Part model, mm, in its own coordinate system. A direction names the side the tool comes from. Coordinates: 2 decimals unless noted, no trailing zeros. Loops run counter-clockwise (first coordinate to the right, second up) from the corner with the lowest first, then second, coordinate; pieces in that order, holes last. Notation, with made-up numbers: (-16, 36.25) -> (30, 36.25) arc R34 cw to (30, 69.25) -> close; hole circle Ø10 at (-26.5, -7.75). An arc over 180 degrees is marked (long way). One line per question, with ' | ' between items. Start each with the question number.
1) Cut at D-D (y = 3.25). List the corners of the cut face in (x, z), plus the area to 3 significant figures.
2) Cut at A-A (z = 10). List the corners of the cut face in (x, y).
3) Drop flat-ended pins along their axis: pin 1 (2 mm diameter, centred on y = 6, z = 5, fed in from -X); pin 2 (3 mm diameter, centred on y = 10.5, z = 5.5, fed in from +X); pin 3 (7.5 mm diameter, centred on y = 10, z = 10, fed in from -X); pin 4 (3 mm diameter, centred on x = 15, z = 10, fed in from +Y). Give the stop position or say it passes through.
4) Cut at C-C (x = 15). List the corners of the cut face in (y, z).
5) 3-axis set-ups, long thin cutter, end or side, ignore diameter. For faces 1 (the face through (9.87, 6.25, 10.05)), 2 (the face through (0.57, 0.6, 3.8)), 3 (the face through (25, 3, 10)), 4 (the face through (0, 12.98, 0.38)), 5 (the face through (16, 7, 4)): which of +Z, -Z, +X, -X, +Y, -Y reach the whole face in a straight line?
6) Cut at B-B (y = 10). List the corners of the cut face in (x, z).
7) Probe L1, parallel to Z at x = 15, y = 1.5; L2, parallel to Y at x = 3.75, z = 10; L3, parallel to X at y = 3, z = 10. List the from-to ranges inside material, lowest first. Write a range as from..to.
8) Two-plate mould, pull along X, no slides. Class faces 6 (the face through (0.57, 0.185, 12.835)), 7 (the face through (12.907, 3.549, 9.047)), 8 (the face through (10, 6, 20)): released by +X, released by -X, zero draft, split by the parting line, or undercut.
from build123d import *

# Parameters (mm, degrees)
AUFSATZ_LINEAR_AUSTRAGEN1_DEPTH      = 20
AUFSATZ_LINEAR_AUSTRAGEN2_DEPTH      = 20
AUFSATZ_LINEAR_AUSTRAGEN3_DEPTH      = 25
SCHNITT_LINEAR_AUSTRAGEN1_DEPTH      = 20
SCHNITT_LINEAR_AUSTRAGEN1_DEPTH_BACK = 20
SKIZZE2_R                            = 2.3
SKIZZE3_R                            = 3.75
SCHNITT_LINEAR_AUSTRAGEN2_DEPTH      = 34.526109228
SKIZZE4_R                            = 2.3
SCHNITT_LINEAR_AUSTRAGEN3_DEPTH      = 20
FASE1_SIZE                           = 0.75
VERRUNDUNG1_R                        = 2
SKIZZE7_R                            = 4.15
SCHNITT_LINEAR_AUSTRAGEN4_DEPTH      = 20
SKIZZE8_R                            = 4.15
SCHNITT_LINEAR_AUSTRAGEN5_DEPTH      = 20
VERRUNDUNG2_R                        = 1


with BuildPart() as part:
    # Skizze1 → Aufsatz-Linear austragen1 (new body)
    with BuildSketch(Plane.XY):
        Polygon((0, 0), (0, 20), (7, 20), (7, 7), (25, 7), (25, 0), align=None)
    extrude(amount=AUFSATZ_LINEAR_AUSTRAGEN1_DEPTH)

    # Skizze5 → Aufsatz-Linear austragen2 (add)
    with BuildSketch(Plane(origin=(0, 0, 0), x_dir=(-1, 0, 0), z_dir=(0, 0, -1))):
        Polygon((0, 6.5), (0, 13.5), (0.75, 12.75), (0.75, 7.25), align=None)
    extrude(amount=-AUFSATZ_LINEAR_AUSTRAGEN2_DEPTH)

    # Skizze6 → Aufsatz-Linear austragen3 (add)
    with BuildSketch(Plane.ZY):
        Polygon((6.5, 0), (13.5, 0), (12.75, -0.75), (7.25, -0.75), align=None)
    extrude(amount=-AUFSATZ_LINEAR_AUSTRAGEN3_DEPTH)

    # Skizze2 → Schnitt-Linear austragen1 (cut, two sides: drawn at the far end of the back side and taken through both)
    with BuildSketch(Plane.ZY.offset(-SCHNITT_LINEAR_AUSTRAGEN1_DEPTH_BACK)):
        with Locations(Location((10, 10, 0), (0, 0, 270))):
            Circle(SKIZZE2_R)
    extrude(amount=SCHNITT_LINEAR_AUSTRAGEN1_DEPTH + SCHNITT_LINEAR_AUSTRAGEN1_DEPTH_BACK, mode=Mode.SUBTRACT)

    # Skizze3 → Schnitt-Linear austragen2 (cut, through all)
    with BuildSketch(Plane(origin=(7, 0, 0), x_dir=(0, 0, -1), z_dir=(1, 0, 0))):
        with Locations((-10, 10)):
            Circle(SKIZZE3_R)
    extrude(amount=SCHNITT_LINEAR_AUSTRAGEN2_DEPTH, mode=Mode.SUBTRACT)

    # Skizze4 → Schnitt-Linear austragen3 (cut)
    with BuildSketch(Plane(origin=(0, 7, 0), x_dir=(1, 0, 0), z_dir=(0, 1, 0))):
        with Locations(Location((15, -10, 0), (0, 0, 258.031254445))):
            Circle(SKIZZE4_R)
    extrude(amount=-SCHNITT_LINEAR_AUSTRAGEN3_DEPTH, mode=Mode.SUBTRACT)

    # Fase1
    fase1_edges = [part.edges().sort_by_distance(p)[0] for p in [
        (0, 20, 10),
        (7, 20, 10),
        (7, 7, 16.125),
        (25, 7, 16.125),
        (25, 0, 16.75),
        (16, 7, 20),
        (7, 13.5, 20),
        (0, 3.25, 0),
        (0, 3.25, 20),
        (3.5, 20, 20),
        (-0.375, 6.875, 20),
        (-0.375, 13.125, 20),
        (-0.75, 10, 20),
        (-0.375, 6.875, 0),
        (-0.75, 10, 0),
        (-0.375, 13.125, 0),
        (0, 16.75, 20),
        (25, 0, 3.25),
        (25, -0.375, 13.125),
        (25, -0.75, 10),
        (25, -0.375, 6.875),
        (12.5, 0, 20),
        (7, 7, 3.875),
        (25, 7, 3.875),
        (25, 6.25, 10),
        (0, 16.75, 0),
        (3.5, 20, 0),
        (7, 13.5, 0),
        (16, 7, 0),
        (25, 3.5, 0),
        (12.5, 0, 0),
        (25, 3.5, 20),
    ]]
    chamfer(fase1_edges, length=FASE1_SIZE)

    # Verrundung1
    verrundung1_edges = [part.edges().sort_by_distance(p)[0] for p in [
        (0, 0, 3.625),
        (0, -0.375, 13.125),
        (0, -0.375, 6.875),
        (0, -0.75, 10),
        (0, 0, 16.375),
    ]]
    fillet(verrundung1_edges, radius=VERRUNDUNG1_R)

    # Skizze7 → Schnitt-Linear austragen4 (cut)
    with BuildSketch(Plane.ZY):
        with Locations((10, 10)):
            Circle(SKIZZE7_R)
    extrude(amount=SCHNITT_LINEAR_AUSTRAGEN4_DEPTH, mode=Mode.SUBTRACT)

    # Skizze8 → Schnitt-Linear austragen5 (cut)
    with BuildSketch(Plane.XZ):
        with Locations((15, 10)):
            Circle(SKIZZE8_R)
    extrude(amount=SCHNITT_LINEAR_AUSTRAGEN5_DEPTH, mode=Mode.SUBTRACT)

    # Verrundung2
    # the kernel refuses this fillet: 1 mm, written as the material it takes off along each edge
    with BuildSketch(Plane(origin=(15, -0.75, 10), x_dir=(-0.259943773458836, 0, -0.9656237541817109), z_dir=(0.9656237541817109, 0, -0.259943773458836))) as verrundung2_piece_1:
        with BuildLine():
            CenterArc((5.118245837, 1), VERRUNDUNG2_R, 194.477512186, 75.522487814)
            Line((4.15, 0.75), (4.130635083, 0.745))
            ThreePointArc((4.130635083, 0.745), (4.13, 0.375), (4.13, 0))
            Line((4.13, 0), (4.15, -0.02))
            Line((4.15, -0.02), (5.118245837, -0.02))
            Line((5.118245837, -0.02), (5.118245837, 0))
        make_face()
    revolve(axis=Axis((15, -0.75, 10), (0, 1, 0)), revolution_arc=149.866548224, mode=Mode.SUBTRACT)
    with BuildSketch(Plane(origin=(15, -0.75, 10), x_dir=(0.259943773458836, 0, -0.9656237541817109), z_dir=(-0.9656237541817109, 0, -0.259943773458836))) as verrundung2_piece_2:
        with BuildLine():
            CenterArc((5.118245837, -1), VERRUNDUNG2_R, 90, 75.522487814)
            Line((4.15, -0.75), (4.130635083, -0.745))
            ThreePointArc((4.130635083, -0.745), (4.13, -0.375), (4.13, 0))
            Line((4.13, 0), (4.15, 0.02))
            Line((4.15, 0.02), (5.118245837, 0.02))
            Line((5.118245837, 0.02), (5.118245837, 0))
        make_face()
    revolve(axis=Axis((15, -0.75, 10), (0, -1, 0)), revolution_arc=149.866548224, mode=Mode.SUBTRACT)
    with BuildSketch(Plane(origin=(-0.75, 10, 10), x_dir=(0, -0.9656237541817109, -0.2599437734588364), z_dir=(0, -0.2599437734588364, 0.9656237541817109))) as verrundung2_piece_3:
        with BuildLine():
            CenterArc((5.118245837, 1), VERRUNDUNG2_R, 194.477512186, 75.522487814)
            Line((4.15, 0.75), (4.130635083, 0.745))
            ThreePointArc((4.130635083, 0.745), (4.13, 0.375), (4.13, 0))
            Line((4.13, 0), (4.15, -0.02))
            Line((4.15, -0.02), (5.118245837, -0.02))
            Line((5.118245837, -0.02), (5.118245837, 0))
        make_face()
    revolve(axis=Axis((-0.75, 10, 10), (1, 0, 0)), revolution_arc=149.866548224, mode=Mode.SUBTRACT)
    with BuildSketch(Plane(origin=(-0.75, 10, 10), x_dir=(0, -0.9656237541817109, 0.2599437734588359), z_dir=(0, -0.2599437734588359, -0.9656237541817109))) as verrundung2_piece_4:
        with BuildLine():
            CenterArc((5.118245837, -1), VERRUNDUNG2_R, 90, 75.522487814)
            Line((4.15, -0.75), (4.130635083, -0.745))
            ThreePointArc((4.130635083, -0.745), (4.13, -0.375), (4.13, 0))
            Line((4.13, 0), (4.15, 0.02))
            Line((4.15, 0.02), (5.118245837, 0.02))
            Line((5.118245837, 0.02), (5.118245837, 0))
        make_face()
    revolve(axis=Axis((-0.75, 10, 10), (-1, 0, 0)), revolution_arc=149.866548224, mode=Mode.SUBTRACT)


solid = part.part
Reported:
1) outline: (0, 0.75) -> (0.75, 0) -> (24.25, 0) -> (25, 0.75) -> (25, 19.25) -> (24.25, 20) -> (0.75, 20) -> (0, 19.25) -> close; hole circle Ø4.6 at (15, 10) | area: 482 mm²
2) outline: (0, 1.25) arc R2 ccw to (2, -0.75) -> (9.88, -0.75) arc R1 ccw to (10.85, 0) -> (12.7, 0) -> (12.7, 6.25) -> (7, 6.25) -> (7, 7.7) -> (0, 7.7) -> close; (0, 12.3) -> (7, 12.3) -> (7, 19.25) -> (6.25, 20) -> (0.75, 20) -> (0, 19.25) -> close; (17.3, 0) -> (19.15, 0) arc R1 ccw to (20.12, -0.75) -> (24.25, -0.75) -> (25, 0) -> (25, 5.5) -> (24.25, 6.25) -> (17.3, 6.25) -> close
3) pin 1: stops at x = -0.5 | pin 2: stops at x = 7 | pin 3: stops at x = 0 | pin 4: passes through
4) outline: (0, 0.75) -> (0.75, 0) -> (6.25, 0) -> (7, 0.75) -> (7, 7.7) -> (0, 7.7) -> close; (0, 12.3) -> (7, 12.3) -> (7, 19.25) -> (6.25, 20) -> (0.75, 20) -> (0, 19.25) -> close
5) face 1: +X, +Y | face 2: -Z, -X, -Y | face 3: +Z, -Z, +X, +Y, -Y | face 4: -Z, -X, +Y | face 5: +Z, -Z, +X, +Y
6) outline: (-0.75, 0.75) -> (0, 0) -> (6.25, 0) -> (7, 0.75) -> (7, 7.7) -> (0, 7.7) -> (0, 5.85) arc R1 ccw to (-0.75, 4.88) -> close; (-0.75, 15.12) arc R1 ccw to (0, 14.15) -> (0, 12.3) -> (7, 12.3) -> (7, 19.25) -> (6.25, 20) -> (0, 20) -> (-0.75, 19.25) -> close
7) L1: z = 0..7.7, 12.3..20 | L2: y = -0.75..7.7, 12.3..20 | L3: x = 0..12.7, 17.3..25
8) face 6: released by -X | face 7: undercut | face 8: zero draft
